Study the drawing (mm; zero at the part's minimum x, y, z) and answer. A direction names the side the tool comes from. Coordinates: 2 decimals unless noted, no trailing zeros. Loops run counter-clockwise (first coordinate to the right, second up) from the corner with the lowest first, then second, coordinate; pieces in that order, holes last. Notation, with made-up numbers: (8.5, 39) -> (32.5, 39) arc R23 cw to (32.5, 71) -> close; hole circle Ø1 at (69.25, 55). An arc over 180 degrees is marked (long way). Answer as CSV lines item,"result".
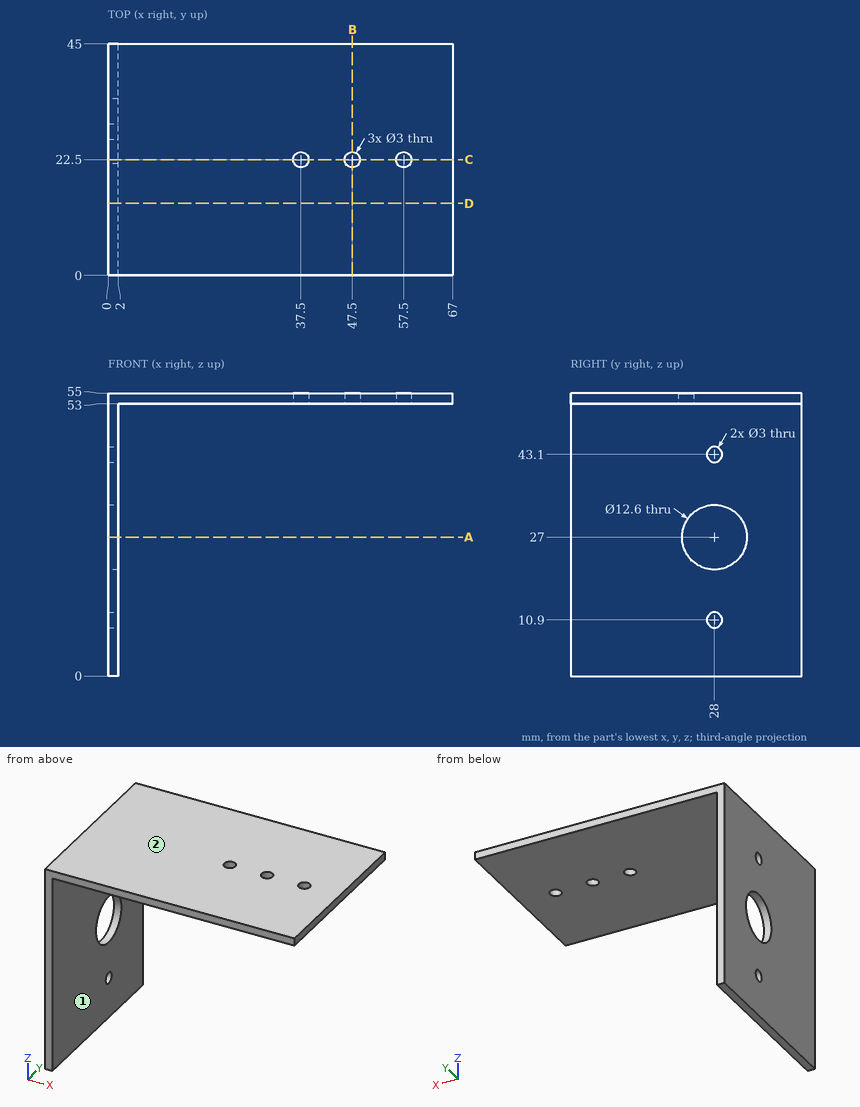
Q1. A cutting plane is placed at C-C, the plane y = 22.5. Write down the section's boundary in (x, z), and give its area (3 significant figures).
Results:
outline,"(0, 0) -> (2, 0) -> (2, 23.93) -> (0, 23.93) -> close; (0, 30.07) -> (2, 30.07) -> (2, 53) -> (36, 53) -> (36, 55) -> (0, 55) -> close; (39, 53) -> (46, 53) -> (46, 55) -> (39, 55) -> close; (49, 53) -> (56, 53) -> (56, 55) -> (49, 55) -> close; (59, 53) -> (67, 53) -> (67, 55) -> (59, 55) -> close"
area,"210 mm²"
Q2. A cutting plane is placed at A-A, the plane z = 27. Write down the section's boundary in (x, y), and give its area (3 significant figures).
Results:
outline,"(0, 0) -> (2, 0) -> (2, 21.7) -> (0, 21.7) -> close; (0, 34.3) -> (2, 34.3) -> (2, 45) -> (0, 45) -> close"
area,"64.8 mm²"
Q3. For the marked faces 1 and 2, determine the directions among +Z, -Z, +X, -X, +Y, -Y from which every point of the face is accessible in a straight line to the end or side of a thin tool.
Results:
face 1,"-Z, +X, +Y, -Y"
face 2,"+Z, +X, -X, +Y, -Y"
Q4. A cutting plane is placed at B-B, the plane x = 47.5. Write down the section's boundary in (y, z), and give its area (3 significant figures).
Results:
outline,"(0, 53) -> (21, 53) -> (21, 55) -> (0, 55) -> close; (24, 53) -> (45, 53) -> (45, 55) -> (24, 55) -> close"
area,"84.0 mm²"
Q5. A cutting plane is placed at D-D, the plane y = 14. Write down the section's boundary in (x, z).
Results:
outline,"(0, 0) -> (2, 0) -> (2, 53) -> (67, 53) -> (67, 55) -> (0, 55) -> close"
Q6. Find the intervals of material crossed by probe 1 along X at (y, z) = (22.5, 54.1); probe 2 along Y at (x, z) = (57.5, 53.85); probe 3 along Y at (x, z) = (0.85, 10.9), in increasing order. Write a range as [from, to].
Results:
probe 1,"x = [0, 36], [39, 46], [49, 56], [59, 67]"
probe 2,"y = [0, 21], [24, 45]"
probe 3,"y = [0, 26.5], [29.5, 45]"
Q7. Given pin 1 Ø4 at (y, z) = (28, 10.9) entering from -X; pin 2 Ø14.5 at (y, z) = (28, 27) entering from +X; pin 3 Ø5 at (x, y) = (58.5, 34) entering from -Z; pin 4 Ø1.8 at (x, y) = (47.5, 22.5) entering from +Z, each flat-ended and moving along its own axis, determine where each tip first touches the part or whether it passes through.
Results:
pin 1,"stops at x = 0"
pin 2,"stops at x = 2"
pin 3,"stops at z = 53"
pin 4,"passes through"
